Can you work these out from the model? Positions are in its coordinate system, mm. Round coordinates to 2 decimals unless told otherwise and drop trailing zeros. Loops run counter-clockwise (first coordinate to the right, second up) from the corner with the lowest first, then second, coordinate; pieces in that order, holes last. Notation, with made-up numbers: (28.5, -38) -> (84.5, -38) arc R7 ccw to (84.5, -33) -> close; hole circle Ø8 at (70.5, 61.5). An arc over 180 degrees is marked (long way). Use a Markdown table: item, result.
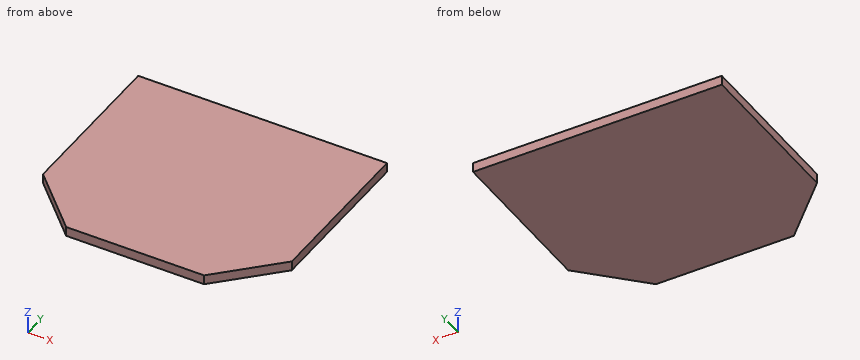
from build123d import *

# Parameters (mm, degrees)
BOSS_EXTRUDE1_DEPTH = 12.7


with BuildPart() as part:
    # Sketch2 → Boss-Extrude1 (new body)
    with BuildSketch(Plane.XY):
        Polygon((0, 0), (183.134, 0), (256.772100193, 73.638100193), (256.772100193, 290.554100193), (-73.638100193, 290.554100193), (-73.638100193, 73.638100193), align=None)
    extrude(amount=BOSS_EXTRUDE1_DEPTH)


solid = part.part
1. I want a section at C-C (y = 61). Please give me the cut outline in (x, z).
Answer sheet:
| item | result |
|---|---|
| outline | (-61, 0) -> (244.13, 0) -> (244.13, 12.7) -> (-61, 12.7) -> close |
2. Will these pins go through, and if not, where does the flat tip stop? pin 1 Ø6 at (x, z) = (-28.5, 4.5) entering from -Y; pin 2 Ø5 at (x, z) = (214.5, 6) entering from -Y; pin 3 Ø2 at (y, z) = (70.5, 6) entering from -X.
Answer sheet:
| item | result |
|---|---|
| pin 1 | stops at y = 25.5 |
| pin 2 | stops at y = 28.87 |
| pin 3 | stops at x = -71.5 |
3. I want a section at A-A (z = 10). Please give me the cut outline in (x, y), plus the area to 3 significant figures.
Answer sheet:
| item | result |
|---|---|
| outline | (-73.64, 73.64) -> (0, 0) -> (183.13, 0) -> (256.77, 73.64) -> (256.77, 290.55) -> (-73.64, 290.55) -> close |
| area | 90,600 mm² |
4. I need wall thicknesses on line 1 (Y direction, x = 187, z = 1.5); line 2 (Y direction, x = -50.5, z = 6.5); line 3 (X direction, y = 71, z = 6.75). Which ranges of each line are inside material? Lowest first, please.
Answer sheet:
| item | result |
|---|---|
| line 1 | y = 3.87 to 290.55 |
| line 2 | y = 50.5 to 290.55 |
| line 3 | x = -71 to 254.13 |
5. I want a section at B-B (x = -23). Please give me the cut outline in (y, z).
Answer sheet:
| item | result |
|---|---|
| outline | (23, 0) -> (290.55, 0) -> (290.55, 12.7) -> (23, 12.7) -> close |
